Verification items for the finished model (mm, model axes). Give positions to 0.01 mm unless a question says otherwise; leave off trailing zeros. Order: outer loops, then holes, each group sorted by start corner. A loop starts at its lowest first (then second) coordinate and runs counter-clockwise, first axis right, second up.
(1) Sectioned sample at A-A on x = -21. Record the cut outline in (y, z), plus the area to 3 significant figures.
(2) Scan lines: L1, parallel to X at y = 1.05, z = -20; L2, parallel to Z at x = -45, y = 0.8; L3, parallel to X at y = 1, z = -19. Record each from-to range of solid material in increasing order.
(3) Sectioned sample at D-D on x = 5.5. Record the cut outline in (y, z), plus the area to 3 significant figures.
(4) Gauge pin test, flat ends, axial feed: pin 1 (0.5 mm diameter, centred on y = 1, z = -18.5, fed in from +X); pin 2 (2.5 mm diameter, centred on x = -45, z = 20, fed in from -Y); pin 3 (0.8 mm diameter, centred on x = 10.5, y = 1, fed in from +Z). Record the tip position at first contact, or that the pin passes through.
(5) Sectioned sample at B-B on y = 1.05. Count the separate pieces of the cut face and the enclosed holes in it, plus the area to 3 significant figures.
(6) Sectioned sample at C-C on z = -5.5. Record the cut outline in (x, y), plus the area to 3 significant figures.
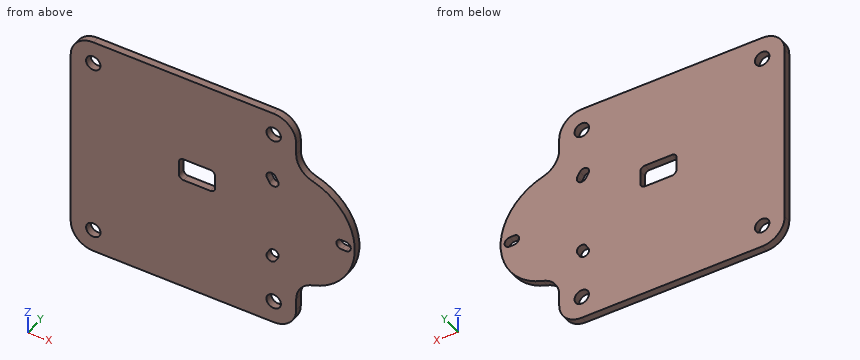
```python
from build123d import *

# Parameters (mm, degrees)
BOSS_EXTRUDE1_DEPTH = 1.6
FILLET1_R           = 5
CUT_EXTRUDE1_DEPTH  = 56.924592086
SKETCH3_R           = 1.6
CUT_EXTRUDE2_DEPTH  = 56.924592086
FILLET2_R           = 5
SKETCH4_W           = 8
SKETCH4_H           = 5
CUT_EXTRUDE3_DEPTH  = 56.924592086
FILLET3_R           = 1


with BuildPart() as part:
    # Sketch1 → Boss-Extrude1 (new body)
    with BuildSketch(Plane(origin=(0, 0, 0), x_dir=(1, 0, 0), z_dir=(0, 1, 0))):
        with BuildLine():
            Line((-50, 25), (-50, -25))
            Line((-50, -25), (0, -25))
            Line((0, -25), (0, -13))
            ThreePointArc((0, -13), (13, 0), (0, 13))
            Line((0, 13), (0, 25))
            Line((0, 25), (-50, 25))
        make_face()
    extrude(amount=BOSS_EXTRUDE1_DEPTH)

    # Fillet1
    fillet1_edges = [part.edges().sort_by_distance(p)[0] for p in [
        (0, 0.8, 25),
        (-50, 0.8, 25),
        (-50, 0.8, -25),
        (0, 0.8, -25),
    ]]
    fillet(fillet1_edges, radius=FILLET1_R)

    # Sketch2 → Cut-Extrude1 (cut, through all)
    with BuildSketch(Plane(origin=(0, 0, 0), x_dir=(1, 0, 0), z_dir=(0, 1, 0))):
        with BuildLine():
            Line((-6.452627944, -8.976279442), (-5.952627944, -8.110254038))
            ThreePointArc((-5.952627944, -8.110254038), (-4.45, -7.707626094), (-4.047372056, -9.210254038))
            Line((-4.047372056, -9.210254038), (-4.547372056, -10.076279442))
            ThreePointArc((-4.547372056, -10.076279442), (-6.05, -10.478907386), (-6.452627944, -8.976279442))
        make_face()
        with BuildLine():
            Line((10, 1.1), (11, 1.1))
            ThreePointArc((11, 1.1), (12.1, 0), (11, -1.1))
            Line((11, -1.1), (10, -1.1))
            ThreePointArc((10, -1.1), (8.9, 0), (10, 1.1))
        make_face()
        with BuildLine():
            Line((-5.952627944, 8.110254038), (-6.452627944, 8.976279442))
            ThreePointArc((-6.452627944, 8.976279442), (-6.05, 10.478907386), (-4.547372056, 10.076279442))
            Line((-4.547372056, 10.076279442), (-4.047372056, 9.210254038))
            ThreePointArc((-4.047372056, 9.210254038), (-4.45, 7.707626094), (-5.952627944, 8.110254038))
        make_face()
    extrude(amount=CUT_EXTRUDE1_DEPTH, mode=Mode.SUBTRACT)

    # Sketch3 → Cut-Extrude2 (cut, through all)
    with BuildSketch(Plane(origin=(0, 0, 0), x_dir=(1, 0, 0), z_dir=(0, 1, 0))):
        with Locations(Location((-45, 20, 0), (0, 0, 270))):
            Circle(SKETCH3_R)
        with Locations(Location((-5, 20, 0), (0, 0, 270))):
            Circle(SKETCH3_R)
        with Locations(Location((-5, -20, 0), (0, 0, 270))):
            Circle(SKETCH3_R)
        with Locations(Location((-45, -20, 0), (0, 0, 270))):
            Circle(SKETCH3_R)
    extrude(amount=CUT_EXTRUDE2_DEPTH, mode=Mode.SUBTRACT)

    # Fillet2
    fillet2_edges = [part.edges().sort_by_distance(p)[0] for p in [
        (0, 0.8, 13),
        (0, 0.8, -13),
    ]]
    fillet(fillet2_edges, radius=FILLET2_R)

    # Sketch4 → Cut-Extrude3 (cut, through all)
    with BuildSketch(Plane.XZ):
        with Locations((-22, 3)):
            Rectangle(SKETCH4_W, SKETCH4_H)
    extrude(amount=-CUT_EXTRUDE3_DEPTH, mode=Mode.SUBTRACT)

    # Fillet3
    fillet3_edges = [part.edges().sort_by_distance(p)[0] for p in [
        (-26, 0.8, 0.5),
        (-26, 0.8, 5.5),
        (-18, 0.8, 5.5),
        (-18, 0.8, 0.5),
    ]]
    fillet(fillet3_edges, radius=FILLET3_R)


solid = part.part
```
Ans:
1. outline: (0, -25) - (1.6, -25) - (1.6, 0.5) - (0, 0.5) - close; (0, 5.5) - (1.6, 5.5) - (1.6, 25) - (0, 25) - close
1. area: 72.0 mm2
2. L1: x = -50 to -46.6, -43.4 to -6.6, -3.4 to 0
2. L2: z = -25 to -21.6, -18.4 to 18.4, 21.6 to 25
2. L3: x = -50 to -46.25, -43.75 to -6.25, -3.75 to 0
3. outline: (0, -11.78) - (1.6, -11.78) - (1.6, 11.78) - (0, 11.78) - close
3. area: 37.7 mm2
4. pin 1: stops at x = 0
4. pin 2: passes through
4. pin 3: stops at z = 8.18
5. separate pieces: 1
5. enclosed holes: 8
5. area: 2,660 mm2
6. outline: (-50, 0) - (11.78, 0) - (11.78, 1.6) - (-50, 1.6) - close
6. area: 98.8 mm2
